from build123d import *

# Parameters (mm, degrees)
DODANIE_WYCI_GNI_CIE1_DEPTH       = 3
WYCI_GNI_CIE_CIENKA_CIANKA2_DEPTH = 2
WYTNIJ_WYCI_GNI_CIE1_DEPTH        = 27
WYTNIJ_WYCI_GNI_CIE1_DEPTH_BACK   = 40
SZKIC3_R                          = 0.75
ZAOKR_GLENIE2_R                   = 1
WYTNIJ_WYCI_GNI_CIE2_DEPTH        = 100.81161788
WYTNIJ_WYCI_GNI_CIE2_DEPTH_BACK   = 0.0001
SZKIC4_W                          = 51
SZKIC4_H                          = 5


with BuildPart() as part:
    # Szkic1 → Dodanie-wyciągnięcie1 (new body)
    with BuildSketch(Plane(origin=(0, 0, 0), x_dir=(1, 0, 0), z_dir=(0, 1, 0))):
        Polygon((-24.742105263, -43.144736842), (36.257894737, -43.144736842), (36.257894737, -81.144736842), (23.757894737, -92.944736842), (-12.242105263, -92.944736842), (-24.742105263, -81.144736842), align=None)
    extrude(amount=DODANIE_WYCI_GNI_CIE1_DEPTH)

    # Szkic2 → Wyciągnięcie-cienka ścianka2 (add)
    with BuildSketch(Plane(origin=(0, 3, 0), x_dir=(1, 0, 0), z_dir=(0, 1, 0))):
        Polygon((23.757894737, -92.944736842), (-12.242105263, -92.944736842), (-24.742105263, -81.144736842), (-24.742105263, -43.144736842), (36.257894737, -43.144736842), (36.257894737, -81.144736842), align=None)
        Polygon((21.770681783, -87.944736842), (-10.25489231, -87.944736842), (-19.742105263, -78.988807814), (-19.742105263, -48.144736842), (31.257894737, -48.144736842), (31.257894737, -78.988807814), align=None, mode=Mode.SUBTRACT)
    extrude(amount=WYCI_GNI_CIE_CIENKA_CIANKA2_DEPTH)

    # Szkic3 → Wytnij-wyciągnięcie1 (cut, two sides: drawn at the far end of the back side and taken through both)
    with BuildSketch(Plane(origin=(0, 5, 0), x_dir=(1, 0, 0), z_dir=(0, 1, 0)).offset(-WYTNIJ_WYCI_GNI_CIE1_DEPTH_BACK)):
        with Locations(Location((0.757894737, -90.444736842, 0), (0, 0, 90))):
            Circle(SZKIC3_R)
        with Locations(Location((10.757894737, -90.444736842, 0), (0, 0, 90))):
            Circle(SZKIC3_R)
        with Locations(Location((-22.242105263, -66.144736842, 0), (0, 0, 90))):
            Circle(SZKIC3_R)
        with Locations(Location((33.757894737, -66.144736842, 0), (0, 0, 90))):
            Circle(SZKIC3_R)
    extrude(amount=WYTNIJ_WYCI_GNI_CIE1_DEPTH + WYTNIJ_WYCI_GNI_CIE1_DEPTH_BACK, mode=Mode.SUBTRACT)

    # Zaokrąglenie2
    # the kernel refuses this fillet: 1 mm, written as the material it takes off along each edge
    with BuildSketch(Plane(origin=(33.757894737, 0, 66.144736842), x_dir=(0, 0, -1), z_dir=(1, 0, 0))) as zaokr_glenie2_piece_1:
        with BuildLine():
            CenterArc((0.75 + ZAOKR_GLENIE2_R, ZAOKR_GLENIE2_R), ZAOKR_GLENIE2_R, 180, 90)
            Line((0.75, ZAOKR_GLENIE2_R), (0.75, 0))
            Line((0.75, 0), (0.75 + ZAOKR_GLENIE2_R, 0))
        make_face()
    revolve(axis=Axis((33.757894737, 0, 66.144736842), (0, 1, 0)), mode=Mode.SUBTRACT)
    with BuildSketch(Plane(origin=(-22.242105263, 0, 66.144736842), x_dir=(0, 0, -1), z_dir=(1, 0, 0))) as zaokr_glenie2_piece_2:
        with BuildLine():
            CenterArc((0.75 + ZAOKR_GLENIE2_R, ZAOKR_GLENIE2_R), ZAOKR_GLENIE2_R, 180, 90)
            Line((0.75, ZAOKR_GLENIE2_R), (0.75, 0))
            Line((0.75, 0), (0.75 + ZAOKR_GLENIE2_R, 0))
        make_face()
    revolve(axis=Axis((-22.242105263, 0, 66.144736842), (0, 1, 0)), mode=Mode.SUBTRACT)
    with BuildSketch(Plane(origin=(-27.242105263, 0, 43.144736842), x_dir=(0, 1, 0), z_dir=(1, 0, 0))) as zaokr_glenie2_piece_3:
        with BuildLine():
            CenterArc((ZAOKR_GLENIE2_R, ZAOKR_GLENIE2_R), ZAOKR_GLENIE2_R, 180, 90)
            Line((0, ZAOKR_GLENIE2_R), (0, 0))
            Line((0, 0), (ZAOKR_GLENIE2_R, 0))
        make_face()
    extrude(amount=66, mode=Mode.SUBTRACT)
    with BuildSketch(Plane(origin=(10.757894737, 0, 90.444736842), x_dir=(0, 0, -1), z_dir=(1, 0, 0))) as zaokr_glenie2_piece_4:
        with BuildLine():
            CenterArc((0.75 + ZAOKR_GLENIE2_R, ZAOKR_GLENIE2_R), ZAOKR_GLENIE2_R, 180, 90)
            Line((0.75, ZAOKR_GLENIE2_R), (0.75, 0))
            Line((0.75, 0), (0.75 + ZAOKR_GLENIE2_R, 0))
        make_face()
    revolve(axis=Axis((10.757894737, 0, 90.444736842), (0, 1, 0)), mode=Mode.SUBTRACT)
    with BuildSketch(Plane(origin=(36.257894737, 0, 40.644736842), x_dir=(0, 1, 0), z_dir=(0, 0, 1)), Plane(origin=(-24.742105263, 0, 83.644736842), x_dir=(0, 1, 0), z_dir=(0, 0, -1))) as zaokr_glenie2_piece_5:
        with BuildLine():
            CenterArc((ZAOKR_GLENIE2_R, ZAOKR_GLENIE2_R), ZAOKR_GLENIE2_R, 180, 90)
            Line((0, ZAOKR_GLENIE2_R), (0, 0))
            Line((0, 0), (ZAOKR_GLENIE2_R, 0))
        make_face()
    extrude(amount=43, mode=Mode.SUBTRACT)
    with BuildSketch(Plane(origin=(0.757894737, 0, 90.444736842), x_dir=(0, 0, -1), z_dir=(1, 0, 0))) as zaokr_glenie2_piece_6:
        with BuildLine():
            CenterArc((0.75 + ZAOKR_GLENIE2_R, ZAOKR_GLENIE2_R), ZAOKR_GLENIE2_R, 180, 90)
            Line((0.75, ZAOKR_GLENIE2_R), (0.75, 0))
            Line((0.75, 0), (0.75 + ZAOKR_GLENIE2_R, 0))
        make_face()
    revolve(axis=Axis((0.757894737, 0, 90.444736842), (0, 1, 0)), mode=Mode.SUBTRACT)
    with BuildSketch(Plane(origin=(38.075830895, 0, 79.428605109), x_dir=(-0.6864526932555783, 0, -0.7271744631944682), z_dir=(-0.7271744631944682, 0, 0.6864526932555782)), Plane(origin=(-10.424169105, 0, 94.660868575), x_dir=(0.686452693255578, 0, -0.7271744631944684), z_dir=(-0.7271744631944684, 0, -0.686452693255578))) as zaokr_glenie2_piece_7:
        with BuildLine():
            CenterArc((ZAOKR_GLENIE2_R, -ZAOKR_GLENIE2_R), ZAOKR_GLENIE2_R, 90, 90)
            Line((0, -ZAOKR_GLENIE2_R), (0, 0))
            Line((0, 0), (ZAOKR_GLENIE2_R, 0))
        make_face()
    extrude(amount=22.18982257, mode=Mode.SUBTRACT)
    with BuildSketch(Plane(origin=(26.257894737, 0, 92.944736842), x_dir=(0, 0, -1), z_dir=(-1, 0, 0))) as zaokr_glenie2_piece_8:
        with BuildLine():
            CenterArc((ZAOKR_GLENIE2_R, -ZAOKR_GLENIE2_R), ZAOKR_GLENIE2_R, 90, 90)
            Line((0, -ZAOKR_GLENIE2_R), (0, 0))
            Line((0, 0), (ZAOKR_GLENIE2_R, 0))
        make_face()
    extrude(amount=41, mode=Mode.SUBTRACT)

    # Szkic4 → Wytnij-wyciągnięcie2 (cut, two sides: drawn at the far end of the back side and taken through both)
    with BuildSketch(Plane(origin=(0, 3, 0), x_dir=(1, 0, 0), z_dir=(0, 1, 0)).offset(-WYTNIJ_WYCI_GNI_CIE2_DEPTH_BACK)):
        with Locations((5.757894737, -45.644736842)):
            Rectangle(SZKIC4_W, SZKIC4_H)
    extrude(amount=WYTNIJ_WYCI_GNI_CIE2_DEPTH + WYTNIJ_WYCI_GNI_CIE2_DEPTH_BACK, mode=Mode.SUBTRACT)


solid = part.part
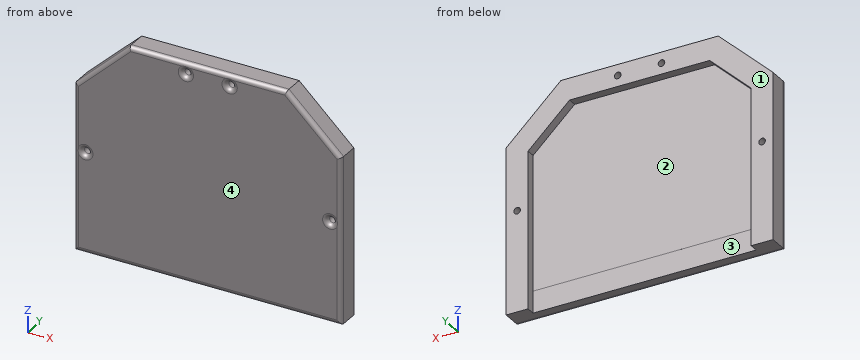
Input: part model. Units: mm. Frame: model coordinates. Face numbers are marked on the shaded views. A direction names the side the tool comes from. Coordinates: 2 decimals unless noted, no trailing zeros. Write each loop counter-clockwise with the first axis right and the second up, starting at its lowest first coordinate (ties: lowest second). Pieces come first, ordered by that corner, then holes. Notation, with made-up numbers: M 30,46 L 50,46 A26 ccw 50,77 Z; hole C 11.25,-5 d3. An arc over 180 degrees is marked long. Answer as a JSON object with one key per item and string values. Group by question number.
(1) Section C-C on z = 80. Output: boundary loops of the cut face in (x, y), plus the area to 3 significant figures.
(2) Section B-B on y = 1.95. Output: boundary loops of the cut face in (x, z), plus the area to 3 significant figures.
(3) Ray query, line 1 along X through (y, z) = (4.7, 47); line 2 along X through (y, z) = (4, 79); line 3 along Y through (x, z) = (21.5, 66.5). Return the intervals inside material, ascending. Write a range as [from, to].
(4) Set-up query: the marked faces 1 and 2. Return all of +Z, -Z, +X, -X, +Y, -Y with unobstructed straight access to the full face (end or side cutting, diameter ignored); none if empty.
(5) Contact query for flat-ended pins moving along their axis: P1, Ø0.9, axis at x = -22.24, z = 66.14, coming from the +Y side; P2, Ø1.6, axis at x = 5, y = 4, coming from the -Z side; P3, Ø4, axis at x = -1.5, z = 45, coming from the +Y side. Output: stop coordinate, or through.
(6) Section A-A on z = 72.5. Output: boundary loops of the cut face in (x, y), plus the area to 3 significant figures.
(7) Mould query, pull axis X, two halves, no side actions, for the marked faces 3 and 4. Classes: pulls with the +X half, pulls with the -X half, needs draft (parallel to the pull), parting line crosses it, or undercut.
Result set:
{
 "1": {"outline": "M -24.74,1 A1 ccw -23.74,0 L 35.26,0 A1 ccw 36.26,1 L 36.26,5 L 30.19,5 L 30.19,3 L -18.67,3 L -18.67,5 L -24.74,5 Z", "area": "207 mm2"},
 "2": {"outline": "M -24.74,43.14 L 36.26,43.14 L 36.26,81.14 L 23.76,92.94 L -12.24,92.94 L -24.74,81.14 Z; hole C -22.24,66.14 d1.5; hole C 0.76,90.44 d1.5; hole C 10.76,90.44 d1.5; hole C 33.76,66.14 d1.5", "area": "2,880 mm2"},
 "3": {"line 1": "x = [-24.74, -19.74], [31.26, 36.26]", "line 2": "x = [-24.74, -19.73], [31.25, 36.26]", "line 3": "y = [0, 3]"},
 "4": {"face 1": "+Z, -Z, +X, -X, +Y", "face 2": "-Z, +Y"},
 "5": {"P1": "passes through", "P2": "stops at z = 87.94", "P3": "stops at y = 3"},
 "6": {"outline": "M -24.74,1 A1 ccw -23.74,0 L 35.26,0 A1 ccw 36.26,1 L 36.26,5 L 31.26,5 L 31.26,3 L -19.74,3 L -19.74,5 L -24.74,5 Z", "area": "203 mm2"},
 "7": {"face 3": "undercut", "face 4": "needs draft"}
}
